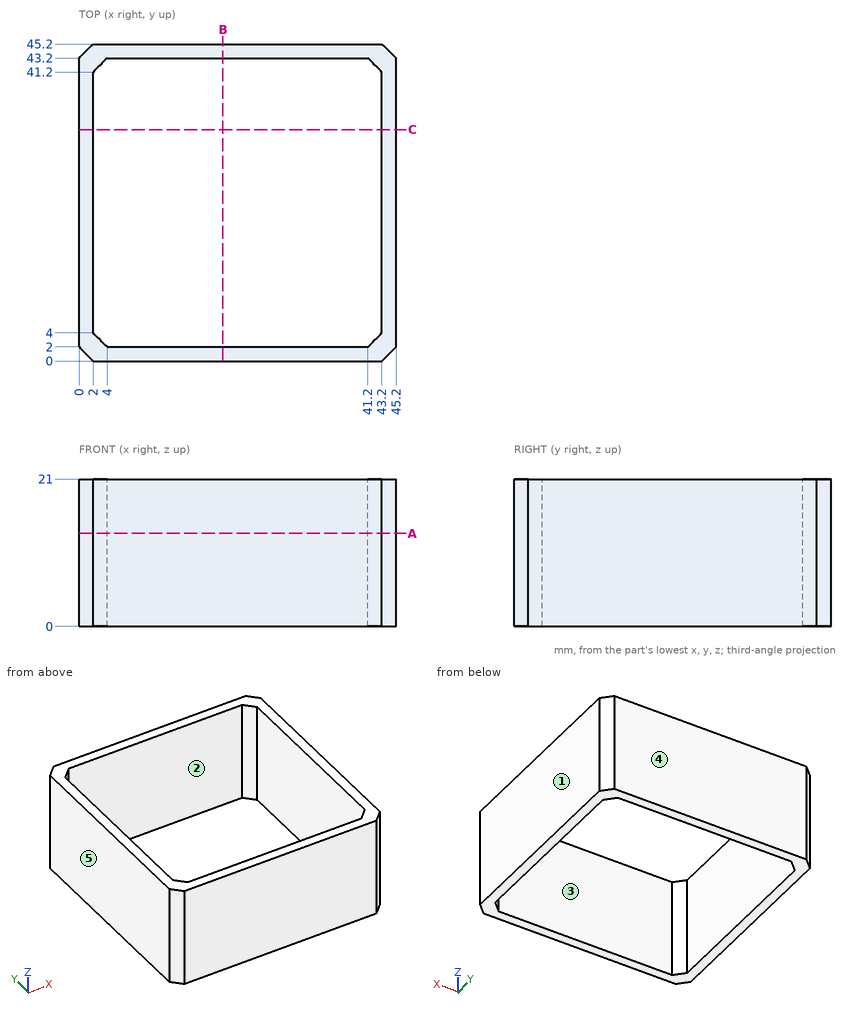
Geometry check sheet. Reference: drawing and pictorial views, mm from the part's lowest x, y, z. A direction names the side the tool comes from. Coordinates: 2 decimals unless noted, no trailing zeros. Order: outer loops, then holes, each group sorted by start corner. A loop starts at its lowest first (then second) coordinate and runs counter-clockwise, first axis right, second up.
Item 1: Tool access check on the marked faces 1 and 2. Record the directions out of +Z, -Z, +X, -X, +Y, -Y that give a thin tool (end or side, any length) a straight path to the whole face; none if there is none.
Item 2: Section check B-B (x = 20.5). Enter the section's corners in (y, z).
Item 3: Section check A-A (z = 13.25). Enter the section's corners in (x, y).
Item 4: Scan lines: line 1 along X through (y, z) = (4, 1); line 2 along Y through (x, z) = (2.5, 16). Record each from-to range of solid material in increasing order.
Item 5: Mould release check, pull along X, two halves, no side actions. Record for the marked faces 3, 4 and 5: released by +X, released by -X, zero draft, split by the parting line, or undercut.
Check sheet entries:
1. face 1: +Z, -Z, +X, +Y, -Y
1. face 2: +Z, -Z
2. outline: (0, 0) - (2, 0) - (2, 21) - (0, 21) - close; (43.2, 0) - (45.2, 0) - (45.2, 21) - (43.2, 21) - close
3. outline: (0, 2) - (2, 0) - (43.2, 0) - (45.2, 2) - (45.2, 43.2) - (43.2, 45.2) - (2, 45.2) - (0, 43.2) - close; hole (2, 4) - (4, 2) - (41.2, 2) - (43.2, 4) - (43.2, 41.2) - (41.2, 43.2) - (4, 43.2) - (2, 41.2) - close
4. line 1: x = 0 to 2, 43.2 to 45.2
4. line 2: y = 0 to 3.5, 41.7 to 45.2
5. face 3: undercut
5. face 4: zero draft
5. face 5: released by -X
